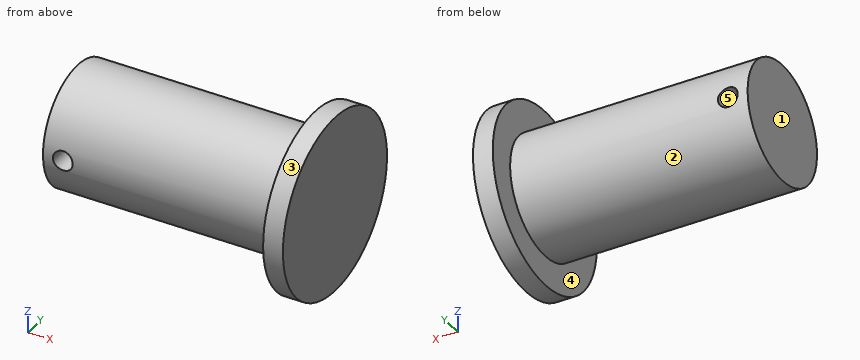
```python
from build123d import *

# Parameters (mm, degrees)
SKETCH1_R               = 15
BOSS_EXTRUDE1_DEPTH     = 30
SKETCH2_R               = 22.5
BOSS_EXTRUDE2_DEPTH     = 5
CUT_EXTRUDE1_DEPTH      = 48.302219821
CUT_EXTRUDE1_DEPTH_BACK = 48.302219821
SKETCH3_R               = 2.5


with BuildPart() as part:
    # Sketch1 → Boss-Extrude1 (new, symmetric)
    with BuildSketch(Plane(origin=(0, 0, 0), x_dir=(0, 0, -1), z_dir=(1, 0, 0))):
        Circle(SKETCH1_R)
    extrude(amount=BOSS_EXTRUDE1_DEPTH, both=True)

    # Sketch2 → Boss-Extrude2 (add)
    with BuildSketch(Plane(origin=(30, 0, 0), x_dir=(0, 0, -1), z_dir=(1, 0, 0))):
        Circle(SKETCH2_R)
    extrude(amount=BOSS_EXTRUDE2_DEPTH)

    # Sketch3 → Cut-Extrude1 (cut, two sides: drawn at the far end of the back side and taken through both)
    with BuildSketch(Plane(origin=(0, 0, 0), x_dir=(1, 0, 0), z_dir=(0, 1, 0)).offset(-CUT_EXTRUDE1_DEPTH_BACK)):
        with Locations(Location((-25, 0, 0), (0, 0, 270))):
            Circle(SKETCH3_R)
    extrude(amount=CUT_EXTRUDE1_DEPTH + CUT_EXTRUDE1_DEPTH_BACK, mode=Mode.SUBTRACT)


solid = part.part
```
Geometry check sheet. Reference: the model listing, model coordinates, mm. Face numbers are marked on the shaded views. A direction names the side the tool comes from. Coordinates: 2 decimals unless noted, no trailing zeros. Loops run counter-clockwise (first coordinate to the right, second up) from the corner with the lowest first, then second, coordinate; pieces in that order, holes last. Notation, with made-up numbers: (51.25, -5.75) -> (96.25, -5.75) arc R25 cw to (96.25, 18.25) -> close; hole circle Ø11 at (59.5, 61.5). An arc over 180 degrees is marked (long way). Put each result on its own line as item: value.
1) Release check for a two-part mould opening along Z. For the marked faces 3, 4 and 5 record: released by +Z, released by -Z, zero draft, split by the parting line, or undercut.
Result set:
face 3: split by the parting line
face 4: zero draft
face 5: undercut
2) Thickness scan on line 1 (X direction, y = 14, z = 17); line 2 (X direction, y = 2.5, z = 0); line 3 (X direction, y = 14, z = -2). Record the ranges inside material, lowest first.
Result set:
line 1: x = 30 to 35
line 2: x = -30 to -27.5, -22.5 to 35
line 3: x = -30 to -26.5, -23.5 to 35
3) Cross-section at B-B on y = 0. Record the boundary of the cut face in (x, z).
Result set:
outline: (-30, -15) -> (30, -15) -> (30, -22.5) -> (35, -22.5) -> (35, 22.5) -> (30, 22.5) -> (30, 15) -> (-30, 15) -> close; hole circle Ø5 at (-25, 0)
4) Gauge pin test, flat ends, axial feed: pin 1 Ø8 at (x, z) = (1, -6.5) entering from +Y; pin 2 Ø4 at (x, z) = (-25, 0) entering from +Y; pin 3 Ø1 at (x, y) = (-10.5, -13.5) entering from -Z; pin 4 Ø8 at (x, z) = (1.5, 4) entering from +Y. Record the tip position at first contact, or that the pin passes through.
Result set:
pin 1: stops at y = 14.79
pin 2: passes through
pin 3: stops at z = -7.48
pin 4: stops at y = 15
5) Tool access check on the marked faces 1 and 2. Record the directions out of +Z, -Z, +X, -X, +Y, -Y that give a thin tool (end or side, any length) a straight path to the whole face; none if there is none.
Result set:
face 1: +Z, -Z, -X, +Y, -Y
face 2: -X
6) Cross-section at A-A on z = 0. Record the boundary of the cut face in (x, y), plus the area to 4 significant figures.
Result set:
outline: (-30, -15) -> (-27.5, -15) -> (-27.5, 15) -> (-30, 15) -> close; (-22.5, -15) -> (30, -15) -> (30, -22.5) -> (35, -22.5) -> (35, 22.5) -> (30, 22.5) -> (30, 15) -> (-22.5, 15) -> close
area: 1,875 mm^2
7) Cross-section at D-D on x = -25. Record the boundary of the cut face in (y, z).
Result set:
outline: (-14.79, -2.5) arc R15 ccw to (14.79, -2.5) -> close; (-14.79, 2.5) -> (14.79, 2.5) arc R15 ccw to start
8) Cross-section at C-C on z = -12. Record the boundary of the cut face in (x, y), plus the area to 3 significant figures.
Result set:
outline: (-30, -9) -> (30, -9) -> (30, -19.03) -> (35, -19.03) -> (35, 19.03) -> (30, 19.03) -> (30, 9) -> (-30, 9) -> close
area: 1,270 mm^2
